Geometry check sheet. Reference: the model listing, model coordinates, mm. Face numbers are marked on the shaded views. A direction names the side the tool comes from. Round coordinates to 2 decimals unless told otherwise and drop trailing zeros. Order: outer loops, then holes, each group sorted by start corner. A loop starts at its lowest first (then second) coordinate and runs counter-clockwise, first axis right, second up. Notation, with made-up numbers: M 69.25,0.5 L 110.25,0.5 A14 ccw 110.25,7.5 Z; hole C 77,70.25 d3. An arc over 180 degrees is marked long. Answer as a JSON object with one key per item and string values. Group by question number.
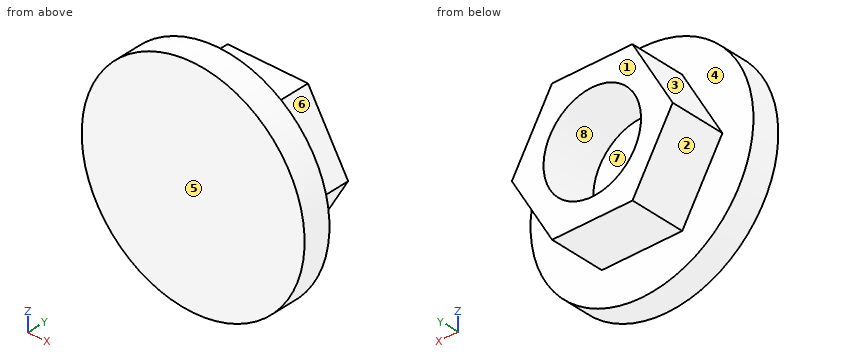
```python
from build123d import *

# Parameters (mm, degrees)
CROQUIS1_R              = 4
SALIENTE_EXTRUIR2_DEPTH = 1
CROQUIS2_R              = 1.75
SALIENTE_EXTRUIR3_DEPTH = 2


with BuildPart() as part:
    # Croquis1 → Saliente-Extruir2 (new body)
    with BuildSketch(Plane(origin=(0, 0, 0), x_dir=(1, 0, 0), z_dir=(0, 1, 0))):
        with Locations(Location((0, 0, 0), (0, 0, 270))):
            Circle(CROQUIS1_R)
    extrude(amount=SALIENTE_EXTRUIR2_DEPTH)

    # Croquis2 → Saliente-Extruir3 (add)
    with BuildSketch(Plane(origin=(0, 1, 0), x_dir=(1, 0, 0), z_dir=(0, 1, 0))):
        Polygon((1.44192427, 2.500837406), (-1.444826589, 2.499161751), (-2.88675086, -0.001675655), (-1.44192427, -2.500837406), (1.444826589, -2.499161751), (2.88675086, 0.001675655), align=None)
        with Locations(Location((0, 0, 0), (0, 0, 270))):
            Circle(CROQUIS2_R, mode=Mode.SUBTRACT)
    extrude(amount=SALIENTE_EXTRUIR3_DEPTH)


solid = part.part
```
1) Sectioned sample at A-A (y = 1.7). Record the boundary of the cut face in (x, z), then the cut area to 3 significant figures.
2) Sectioned sample at D-D (y = 0.8). Record the boundary of the cut face in (x, z).
3) Thickness scan on line 1 along Y through (x, z) = (3, 0.25); line 2 along X through (y, z) = (2.85, -1.5); line 3 along X through (y, z) = (1.7, -1). Record the ranges inside material, lowest first. Write a range as [from, to].
4) Sectioned sample at B-B (x = 0). Record the boundary of the cut face in (y, z), then the cut area to 3 significant figures.
5) Set-up check for the marked faces 1, 2, 3 and 4: record each of +Z, -Z, +X, -X, +Y, -Y from which the full face is reachable in a straight line by a thin tool's end or side.
6) Go/stop test with flat-tipped pins: P1, Ø1, axis at x = 1, y = 2.5, coming from the +Z side; P2, Ø1, axis at y = 1, z = -2, coming from the -X side; P3, Ø2, axis at x = 0.5, z = -0.5, coming from the +Y side. Record where each tip stops, or that it passes through.
7) Release check for a two-part mould opening along Z. For the marked faces 5, 6, 7 and 8 record: +Z half, -Z half, draft (parallel to the pull), parting line (faces both ways), or undercut.
8) Sectioned sample at C-C (z = -0.25). Record the boundary of the cut face in (x, y), then the cut area to 3 significant figures.
Final values:
{
 "1": {"outline": "M -2.89,0 L -1.44,-2.5 L 1.44,-2.5 L 2.89,0 L 1.44,2.5 L -1.44,2.5 Z; hole C 0,0 d3.5", "area": "12.0 mm^2"},
 "2": {"outline": "C 0,0 d8"},
 "3": {"line 1": "y = [0, 1]", "line 2": "x = [-2.02, -0.9], [0.9, 2.02]", "line 3": "x = [-2.31, -1.44], [1.44, 2.31]"},
 "4": {"outline": "M 0,-4 L 1,-4 L 1,-2.5 L 3,-2.5 L 3,-1.75 L 1,-1.75 L 1,1.75 L 3,1.75 L 3,2.5 L 1,2.5 L 1,4 L 0,4 Z", "area": "11.0 mm^2"},
 "5": {"face 1": "+Z, -Z, +X, -X, +Y", "face 2": "-Z, -X, +Y", "face 3": "+Z, -X, +Y", "face 4": "+Y"},
 "6": {"P1": "stops at z = 2.5", "P2": "stops at x = -3.71", "P3": "stops at y = 1"},
 "7": {"face 5": "draft", "face 6": "+Z half", "face 7": "undercut", "face 8": "undercut"},
 "8": {"outline": "M -3.99,0 L 3.99,0 L 3.99,1 L 2.74,1 L 2.74,3 L 1.73,3 L 1.73,1 L -1.73,1 L -1.73,3 L -2.74,3 L -2.74,1 L -3.99,1 Z", "area": "12.0 mm^2"}
}
